Autodesk Inventor part; units mm, degrees
ref_plane "1_XY" through (18.7452, 0, 0) normal (1, 0, 0) x (0, 0, -1)
ref_plane "1_YZ" through (18.7452, 0, 0) normal (0, 0, -1) x (0, 1, 0)
ref_plane "1_ZX" through (18.7452, 0, 0) normal (0, 1, 0) x (1, 0, 0)
sketch "Sketch_8" plane through (0, 0, 0) normal (0, 0, 1) x (1, 0, 0)
  line L0 (17.4752, 0) -> (0, 0)
  line L1 (0, 0) -> (0, 4.9085)
  line L2 (0, 4.9085) -> (0.762, 5.6706)
  line L3 (0.762, 5.6706) -> (3.7592, 5.6706)
  line L4 (3.7592, 5.6706) -> (4.2672, 5.1626)
  line L5 (4.2672, 5.1626) -> (4.7752, 5.1626)
  line L6 (4.7752, 5.1626) -> (4.7752, 6.1659)
  line L7 (4.7752, 6.1659) -> (7.9502, 6.1659)
  line L8 (7.9502, 6.1659) -> (7.9502, 8.6106)
  line L9 (7.9502, 8.6106) -> (8.7122, 9.3726)
  line L10 (8.7122, 9.3726) -> (16.7132, 9.3726)
  line L11 (16.7132, 9.3726) -> (17.4752, 8.6106)
  line L12 (17.4752, 8.6106) -> (17.4752, 0)
  line L13 (17.4752, 0) -> (0, 0)
revolve "Revolution1" add sketch "Sketch_8" angle 360 about axis through (17.4752, 0, 0) along (1, 0, 0)
sketch "Sketch_15" plane through (0, 0, 0) normal (0, 0, 1) x (1, 0, 0)
  line L0 (30.1752, 0) -> (17.4752, 0)
  line L1 (17.4752, 0) -> (17.4752, 5.5245)
  line L2 (17.4752, 5.5245) -> (18.7452, 5.5245)
  line L3 (18.7452, 5.5245) -> (18.7452, 5.3721)
  arc A0 (18.7452, 5.3721) -> (19.5453, 4.572) centre (19.5453, 5.3721) ccw
  line L4 (19.5453, 4.572) -> (20.7137, 4.572)
  arc A1 (20.7137, 4.572) -> (21.2166, 4.7498) centre (20.7137, 5.3721) ccw
  line L5 (21.2166, 4.7498) -> (21.2795, 4.8006)
  line L6 (21.2795, 4.8006) -> (22.0351, 5.5563)
  line L7 (22.0351, 5.5563) -> (29.4196, 5.5563)
  line L8 (29.4196, 5.5563) -> (30.1752, 4.8006)
  line L9 (30.1752, 4.8006) -> (30.1752, 0)
  line L10 (30.1752, 0) -> (17.4752, 0)
revolve "Revolution2" add sketch "Sketch_15" angle 360 about axis through (30.1752, 0, 0) along (1, 0, 0)
thread "Thread1"
sketch "Sketch_9" plane through (30.1752, 0, 0) normal (1, 0, 0) x (0, 0, -1)
  line L0 (-18.7452, -37.4904) -> (18.7452, -37.4904)
  line L1 (18.7452, -37.4904) -> (18.7452, 37.4904)
  line L2 (18.7452, 37.4904) -> (-18.7452, 37.4904)
  line L3 (-18.7452, 37.4904) -> (-18.7452, -37.4904)
  line L4 (-3.9306, -18.7452) -> (3.9306, -18.7452)
  line L5 (3.9306, -18.7452) -> (3.9306, 18.7452)
  line L6 (3.9306, 18.7452) -> (-3.9306, 18.7452)
  line L7 (-3.9306, 18.7452) -> (-3.9306, -18.7452)
extrude "Extrusion1" cut sketch "Sketch_9" against normal blind 12.7
sketch "Sketch4" plane through (0, 0, 0) normal (-1, 0, 0) x (0, 0, 1)
  point P0 (0, 0)
hole "Hole1" at (0, 0, 0) direction (1, 0, 0) diameter 4.7625 depth 17.4625 tip angle 120
sketch "Sketch_16" plane through (0, 0, 0) normal (0, 1, 0) x (-1, 0, 0)
  line L0 (-12.7, 9.3726) -> (-12.7, 0)
  line L1 (-12.7, 0) -> (-14.6837, 0)
  line L2 (-14.6837, 0) -> (-14.6837, 7.9273)
  line L3 (-14.6837, 7.9273) -> (-15.113, 8.3566)
  line L4 (-15.113, 8.3566) -> (-16.6624, 8.3566)
  line L5 (-16.6624, 8.3566) -> (-16.6624, 9.3726)
  line L6 (-16.6624, 9.3726) -> (-12.7, 9.3726)
  line L7 (-12.7, 9.3726) -> (-12.7, 0)
revolve "Revolution3" cut sketch "Sketch_16" angle 360 about axis through (12.7, 0, 9.3726) along (0, 0, 1)
thread "Thread2"
sketch "Sketch_24" plane through (0, 0, 0) normal (0, 0, 1) x (1, 0, 0)
  line L0 (4.7752, 0) -> (4.2672, 0)
  line L1 (4.0665, 6.0817) -> (4.6636, 5.4846)
  arc A0 (4.6636, 5.305) -> (4.6636, 5.4846) centre (4.5738, 5.3948) ccw
  line L2 (4.6636, 5.305) -> (4.5212, 5.1626)
  line L3 (4.5212, 5.1626) -> (4.2672, 5.1626)
  line L4 (4.2672, 5.1626) -> (4.2672, 4.9085)
  line L5 (4.2672, 4.9085) -> (4.7752, 4.9085)
  line L6 (4.7752, 4.9085) -> (4.7752, 5.6603)
  line L7 (4.7752, 5.6603) -> (4.2697, 6.1659)
  line L8 (4.2697, 6.1659) -> (4.0665, 6.1659)
  line L9 (4.0665, 6.1659) -> (4.0665, 6.0817)
revolve "Revolution4" add sketch "Sketch_24" angle 360 about axis through (4.7752, 0, 0) along (1, 0, 0)
sketch "Sketch_43" plane through (0, 0, 0) normal (0, 0, 1) x (1, 0, 0)
  circle A0 centre (23.8252, 0) radius 2.0193
extrude "Extrusion2" cut sketch "Sketch_43" along normal mid plane 11.7919
ref_plane "1_XY" through (18.7452, 0, 0) normal (1, 0, 0) x (0, 0, -1)
ref_plane "1_YZ" through (18.7452, 0, 0) normal (0, 0, -1) x (0, 1, 0)
ref_plane "1_ZX" through (18.7452, 0, 0) normal (0, 1, 0) x (1, 0, 0)
ref_plane "c1_XY" through (17.4752, 5.5245, 0) normal (0, 0, 1) x (1, 0, 0)
ref_plane "c1_YZ" through (17.4752, 5.5245, 0) normal (1, 0, 0) x (0, 1, 0)
ref_plane "c1_ZX" through (17.4752, 5.5245, 0) normal (0, 1, 0) x (0, 0, 1)
ref_plane "c2_XY" through (17.4752, -5.5245, 0) normal (0, 0, 1) x (1, 0, 0)
ref_plane "c2_YZ" through (17.4752, -5.5245, 0) normal (1, 0, 0) x (0, 1, 0)
ref_plane "c2_ZX" through (17.4752, -5.5245, 0) normal (0, 1, 0) x (0, 0, 1)
ref_plane "cc1_XY" through (17.4752, 0, 0) normal (0, 0, 1) x (1, 0, 0)
ref_plane "cc1_YZ" through (17.4752, 0, 0) normal (1, 0, 0) x (0, 1, 0)
ref_plane "cc1_ZX" through (17.4752, 0, 0) normal (0, 1, 0) x (0, 0, 1)
ref_plane "cc2_XY" through (18.7452, 0, 0) normal (0, 0, 1) x (1, 0, 0)
ref_plane "cc2_YZ" through (18.7452, 0, 0) normal (1, 0, 0) x (0, 1, 0)
ref_plane "cc2_ZX" through (18.7452, 0, 0) normal (0, 1, 0) x (0, 0, 1)
ref_plane "lovra1_XY" through (25.4, 0, 0) normal (1, 0, 0) x (0, 0, -1)
ref_plane "lovra1_YZ" through (25.4, 0, 0) normal (0, 0, -1) x (0, 1, 0)
ref_plane "lovra1_ZX" through (25.4, 0, 0) normal (0, 1, 0) x (1, 0, 0)
ref_plane "lovra2_XY" through (25.4, 4.699, 0) normal (1, 0, 0) x (0, 0, -1)
ref_plane "lovra2_YZ" through (25.4, 4.699, 0) normal (0, 0, -1) x (0, 1, 0)
ref_plane "lovra2_ZX" through (25.4, 4.699, 0) normal (0, 1, 0) x (1, 0, 0)
ref_plane "lovra21_XY" through (0, 0, 5.2705) normal (1, 0, 0) x (0, 0, -1)
ref_plane "lovra21_YZ" through (0, 0, 5.2705) normal (0, 0, -1) x (0, 1, 0)
ref_plane "lovra21_ZX" through (0, 0, 5.2705) normal (0, 1, 0) x (1, 0, 0)
ref_plane "lovra22_XY" through (0, 0, -5.2705) normal (1, 0, 0) x (0, 0, -1)
ref_plane "lovra22_YZ" through (0, 0, -5.2705) normal (0, 0, -1) x (0, 1, 0)
ref_plane "lovra22_ZX" through (0, 0, -5.2705) normal (0, 1, 0) x (1, 0, 0)
ref_plane "lovra3_XY" through (25.4, -4.699, 0) normal (1, 0, 0) x (0, 0, -1)
ref_plane "lovra3_YZ" through (25.4, -4.699, 0) normal (0, 0, -1) x (0, 1, 0)
ref_plane "lovra3_ZX" through (25.4, -4.699, 0) normal (0, 1, 0) x (1, 0, 0)
ref_plane "olen_XY" through (23.8252, 0, 0) normal (1, 0, 0) x (0, 0, -1)
ref_plane "olen_YZ" through (23.8252, 0, 0) normal (0, 0, -1) x (0, 1, 0)
ref_plane "olen_ZX" through (23.8252, 0, 0) normal (0, 1, 0) x (1, 0, 0)
ref_plane "p1_XY" through (30.1752, 0, 3.9306) normal (1, 0, 0) x (0, 0, -1)
ref_plane "p1_YZ" through (30.1752, 0, 3.9306) normal (0, 0, -1) x (0, 1, 0)
ref_plane "p1_ZX" through (30.1752, 0, 3.9306) normal (0, 1, 0) x (1, 0, 0)
ref_plane "p2_XY" through (30.1752, 0, -3.9306) normal (1, 0, 0) x (0, 0, -1)
ref_plane "p2_YZ" through (30.1752, 0, -3.9306) normal (0, 0, -1) x (0, 1, 0)
ref_plane "p2_ZX" through (30.1752, 0, -3.9306) normal (0, 1, 0) x (1, 0, 0)
ref_plane "port_XY" through (12.7, 0, 0) normal (0, 0, 1) x (1, 0, 0)
ref_plane "port_YZ" through (12.7, 0, 0) normal (1, 0, 0) x (0, 1, 0)
ref_plane "port_ZX" through (12.7, 0, 0) normal (0, 1, 0) x (0, 0, 1)
ref_plane "port2_XY" through (30.1752, 0, 0) normal (1, 0, 0) x (0, 0, -1)
ref_plane "port2_YZ" through (30.1752, 0, 0) normal (0, 0, -1) x (0, 1, 0)
ref_plane "port2_ZX" through (30.1752, 0, 0) normal (0, 1, 0) x (1, 0, 0)
ref_plane "thd1_XY" through (30.1752, 0, 5.5563) normal (1, 0, 0) x (0, 0, -1)
ref_plane "thd1_YZ" through (30.1752, 0, 5.5563) normal (0, 0, -1) x (0, 1, 0)
ref_plane "thd1_ZX" through (30.1752, 0, 5.5563) normal (0, 1, 0) x (1, 0, 0)
ref_plane "thd2_XY" through (30.1752, 0, -5.5563) normal (1, 0, 0) x (0, 0, -1)
ref_plane "thd2_YZ" through (30.1752, 0, -5.5563) normal (0, 0, -1) x (0, 1, 0)
ref_plane "thd2_ZX" through (30.1752, 0, -5.5563) normal (0, 1, 0) x (1, 0, 0)
ref_plane "to_mounting_bracket_XY" through (17.4752, 0, 0) normal (1, 0, 0) x (0, 0, -1)
ref_plane "to_mounting_bracket_YZ" through (17.4752, 0, 0) normal (0, 0, -1) x (0, 1, 0)
ref_plane "to_mounting_bracket_ZX" through (17.4752, 0, 0) normal (0, 1, 0) x (1, 0, 0)
ref_plane "to_nut_XY" through (18.7452, 0, 0) normal (1, 0, 0) x (0, 0, -1)
ref_plane "to_nut_YZ" through (18.7452, 0, 0) normal (0, 0, -1) x (0, 1, 0)
ref_plane "to_nut_ZX" through (18.7452, 0, 0) normal (0, 1, 0) x (1, 0, 0)
ref_plane "to_pin_XY" through (23.8252, 0, 0) normal (0, 0, 1) x (1, 0, 0)
ref_plane "to_pin_YZ" through (23.8252, 0, 0) normal (1, 0, 0) x (0, 1, 0)
ref_plane "to_pin_ZX" through (23.8252, 0, 0) normal (0, 1, 0) x (0, 0, 1)
ref_plane "to_screw_XY" through (12.7, 0, 0) normal (0, 1, 0) x (1, 0, 0)
ref_plane "to_screw_YZ" through (12.7, 0, 0) normal (1, 0, 0) x (0, 0, -1)
ref_plane "to_screw_ZX" through (12.7, 0, 0) normal (0, 0, -1) x (0, 1, 0)
ref_plane "to_tube_XY" through (4.2672, 0, 0) normal (1, 0, 0) x (0, 0, -1)
ref_plane "to_tube_YZ" through (4.2672, 0, 0) normal (0, 0, -1) x (0, 1, 0)
ref_plane "to_tube_ZX" through (4.2672, 0, 0) normal (0, 1, 0) x (1, 0, 0)
properties part number "01P1000_rear_head"
The listing builds one solid part. Answer for the finished solid, in the listing's coordinates (mm). A direction names the side the tool comes from. Coordinates: 2 decimals unless noted, no trailing zeros. Order: outer loops, then holes, each group sorted by start corner. A loop starts at its lowest first (then second) coordinate and runs counter-clockwise, first axis right, second up. Notation, with made-up numbers: M 27.25,22 L 45.25,22 A24 cw 45.25,54 Z; hole C -20,87 d3. An arc over 180 degrees is marked long. Answer as a JSON object with one key per item and string values. Group by question number.
1. Section B-B on y = 1.5 is taken. State how many separate pieces and enclosed holes the cut face has, then the cut area to 3 significant figures.
2. Flat-ended cylindrical pins translate along their axes: P1, Ø1.5, axis at y = -3, z = 3, coming from the -X side; P2, Ø4, axis at x = 21.5, y = -1.5, coming from the +Z side; P3, Ø8.5, axis at x = 24.5, y = -1, coming from the -Z side; P4, Ø6.5, axis at x = 12.7, y = 0, coming from the +Z side. Find the tip coordinate at first contact, or state that the pin passes through.
3. A tool of negligible diameter and unlimited length cuts with its end or side. For faces 5 (the conical face through (21.41, -4.93, 0.07)), 6 (the flat face through (25, 2, -3.931)), 7 (the cylindrical face through (20.14, 4.57, -0.07)), from which of +Z, -Z, +X, -X, +Y, -Y can it reach the whole face along a straight path? Write none if from no direction.
4. Section A-A on x = 12.7 is taken. Write down the section's boundary in (y, z), then the cut area to 3 significant figures.
5. Straight lines are drawn through the part: line 1 (Z direction, x = 9, y = 1.5); line 2 (X direction, y = -4, z = 6.75); line 3 (Y direction, x = 22, z = 1). For each, find the intervals that lie inside material, in ascending order.
6. Determine the mould class of faces 1 (the flat face through (11, -2, 8.357)), 2 (the flat face through (17.475, 6, 0)), 3 (the cylindrical face through (8.85, -0.1, -2.38)), 4 (the cylindrical face through (25.779, -5.556, 0.061)) for opening direction Y: released by +Y, released by -Y, zero draft, split by the parting line, or undercut.
Values follow:
{
 "1": {"separate pieces": "3", "enclosed holes": "0", "area": "253 mm2"},
 "2": {"P1": "x = 0", "P2": "z = 3.93", "P3": "z = -3.93", "P4": "z = 8.36"},
 "3": {"face 5": "-Y", "face 6": "-Z, +X, +Y, -Y", "face 7": "+Y"},
 "4": {"outline": "M -3.96,8.36 L -3.96,8.49 A9.37 ccw long 3.96,8.49 L 3.96,8.36 L 2.41,8.36 L 1.98,7.93 L 1.98,1.32 A2.38 cw long -1.98,1.32 L -1.98,7.93 L -2.41,8.36 Z", "area": "227 mm2"},
 "5": {"line 1": "-9.25 to -1.85, 1.85 to 9.25", "line 2": "7.95 to 17.48", "line 3": "-5.43 to -0.86, 0.86 to 5.43"},
 "6": {"face 1": "undercut", "face 2": "zero draft", "face 3": "undercut", "face 4": "released by -Y"}
}
